Input: part model. Units: mm. Frame: model coordinates. Give positions to 0.01 mm unless a question says otherwise; leave off trailing zeros. Write each loop counter-clockwise with the first axis right and the second up, starting at its lowest first coordinate (ties: lowest second). Pieces come first, ordered by that corner, then holes.
```python
from build123d import *

# Parameters (mm, degrees)
SKETCH_2_W      = 65
SKETCH_2_H      = 105
SKETCH_2_R      = 1.6
EXTRUDE_1_DEPTH = 3
FILLET_1_R      = 5
CHAMFER_1_SIZE  = 1.5


with BuildPart() as part:
    # ｽｹｯﾁ2 → ﾎﾞｽ - 押し出し1 (new body)
    with BuildSketch(Plane.XY):
        Rectangle(SKETCH_2_W, SKETCH_2_H)
        with Locations((-13, 43.5)):
            Circle(SKETCH_2_R, mode=Mode.SUBTRACT)
        with Locations((13, 17.5)):
            Circle(SKETCH_2_R, mode=Mode.SUBTRACT)
        with Locations((13, 43.5)):
            Circle(SKETCH_2_R, mode=Mode.SUBTRACT)
        with Locations((-13, 17.5)):
            Circle(SKETCH_2_R, mode=Mode.SUBTRACT)
        with Locations((-13, -17.5)):
            Circle(SKETCH_2_R, mode=Mode.SUBTRACT)
        with Locations((13, -17.5)):
            Circle(SKETCH_2_R, mode=Mode.SUBTRACT)
        with Locations((-13, -43.5)):
            Circle(SKETCH_2_R, mode=Mode.SUBTRACT)
        with Locations((13, -43.5)):
            Circle(SKETCH_2_R, mode=Mode.SUBTRACT)
        with Locations((-25, 45)):
            Circle(SKETCH_2_R, mode=Mode.SUBTRACT)
        with Locations((25, 45)):
            Circle(SKETCH_2_R, mode=Mode.SUBTRACT)
        with Locations((25, -45)):
            Circle(SKETCH_2_R, mode=Mode.SUBTRACT)
        with Locations((-25, -45)):
            Circle(SKETCH_2_R, mode=Mode.SUBTRACT)
    extrude(amount=EXTRUDE_1_DEPTH)

    # ﾌｨﾚｯﾄ1
    fillet_1_edges = [part.edges().sort_by_distance(p)[0] for p in [
        (32.5, -52.5, 1.5),
        (-32.5, -52.5, 1.5),
        (-32.5, 52.5, 1.5),
        (32.5, 52.5, 1.5),
    ]]
    fillet(fillet_1_edges, radius=FILLET_1_R)

    # 面取り1
    chamfer_1_edges = [part.edges().sort_by_distance(p)[0] for p in [
        (11.4, 17.5, 3),
        (-14.6, 43.5, 3),
        (11.4, 43.5, 3),
        (-14.6, 17.5, 3),
        (-14.6, -17.5, 3),
        (11.4, -17.5, 3),
        (-14.6, -43.5, 3),
        (11.4, -43.5, 3),
    ]]
    chamfer(chamfer_1_edges, length=CHAMFER_1_SIZE)


solid = part.part
```
Item 1: Ray query, line 1 (Y direction, x = 25, z = 2.2); line 2 (Y direction, x = 13, z = 1.05); line 3 (Y direction, x = 13.5, z = 0.55). Return the intervals inside material, ascending.
Item 2: Section C-C (z = 2.4). Give the number of separate pieces and of enclosed holes in the cut face, and give its area (3 significant figures).
Item 3: Pin query (flat end, axial travel): pin 1 (4 mm diameter, centred on x = 13, y = 17.5, fed in from +Z); pin 2 (3.5 mm diameter, centred on x = 13, y = 43.5, fed in from +Z). Return the tip coordinate at first contact, or that it passes through.
Item 4: Section B-B (y = 17.5). Return loops of the section in (x, z), and give its area (3 significant figures).
Item 5: Section A-A (x = -25). Return loops of the section in (y, z), and give its area (3 significant figures).
Solved:
1. line 1: y = -52.5 to -46.6, -43.4 to 43.4, 46.6 to 52.5
1. line 2: y = -52.5 to -45.1, -41.9 to -19.1, -15.9 to 15.9, 19.1 to 41.9, 45.1 to 52.5
1. line 3: y = -52.5 to -45.02, -41.98 to -19.02, -15.98 to 15.98, 19.02 to 41.98, 45.02 to 52.5
2. separate pieces: 1
2. enclosed holes: 12
2. area: 6,610 mm2
3. pin 1: stops at z = 1.9
3. pin 2: stops at z = 1.65
4. outline: (-32.5, 0) - (-14.6, 0) - (-14.6, 1.5) - (-16.1, 3) - (-32.5, 3) - close; (-11.4, 0) - (11.4, 0) - (11.4, 1.5) - (9.9, 3) - (-9.9, 3) - (-11.4, 1.5) - close; (14.6, 0) - (32.5, 0) - (32.5, 3) - (16.1, 3) - (14.6, 1.5) - close
4. area: 171 mm2
5. outline: (-52.5, 0) - (-46.6, 0) - (-46.6, 3) - (-52.5, 3) - close; (-43.4, 0) - (43.4, 0) - (43.4, 3) - (-43.4, 3) - close; (46.6, 0) - (52.5, 0) - (52.5, 3) - (46.6, 3) - close
5. area: 296 mm2
